```python
from build123d import *

# Parameters (mm, degrees)
F0_W     = 50.4226610065
F0_H     = 49.5728440583
F1_DEPTH = 10
F2_T     = -5
F3_W     = 10.1061211899
F3_H     = 5
F4_DEPTH = 0.5
F7_D     = 1
F7_DEPTH = 2
F7_TIP   = 0.3004303095
F8_R     = 5
F9_R     = 5


# Not quite as in the source:
# - a feature names something its author has since deleted; it is built from what else it names


with BuildPart() as f1:
    # F0 (on Top) → F1 (new body)
    with BuildSketch(Plane.XY):
        Rectangle(F0_W, F0_H)
    extrude(amount=F1_DEPTH)

    # F2
    f2_openings = [f1.faces().sort_by_distance(p)[0] for p in [
        (0, 0, 0),
    ]]
    offset(amount=F2_T, openings=f2_openings)

    # F3 (on face) → F4 (cut)
    with BuildSketch(Plane(origin=(0, 0, 0), x_dir=(1, 0, 0), z_dir=(0, 0, -1))):
        with Locations((-12.4224121682, 22.2864220291)):
            Rectangle(F3_W, F3_H)
    extrude(amount=-F4_DEPTH, mode=Mode.SUBTRACT)

    # F7
    with Locations(Plane(origin=(0, 0, 0.5), x_dir=(1, 0, 0), z_dir=(0, 0, -1))):
        with Locations((-12.5449625775, 22.3620422184)):
            Hole(F7_D / 2, depth=F7_DEPTH)
            with Locations((0, 0, -(F7_DEPTH + F7_TIP / 2))):  # 118° drill point
                Cone(0, F7_D / 2, F7_TIP, mode=Mode.SUBTRACT)

    # F8
    f8_edges = [f1.edges().sort_by_distance(p)[0] for p in [
        (-25.211331, -24.786422, 5),
        (25.211331, -24.786422, 5),
        (25.211331, 24.786422, 5),
        (-25.211331, 24.786422, 5),
    ]]
    fillet(f8_edges, radius=F8_R)

    # F9
    f9_edges = [f1.edges().sort_by_distance(p)[0] for p in [
        (25.211331, 0, 10),
        (23.746864, -23.321956, 10),
        (23.746864, 23.321956, 10),
        (0, -24.786422, 10),
        (0, 24.786422, 10),
        (-23.746864, -23.321956, 10),
        (-23.746864, 23.321956, 10),
        (-25.211331, 0, 10),
    ]]
    fillet(f9_edges, radius=F9_R)


solid = f1.part
```
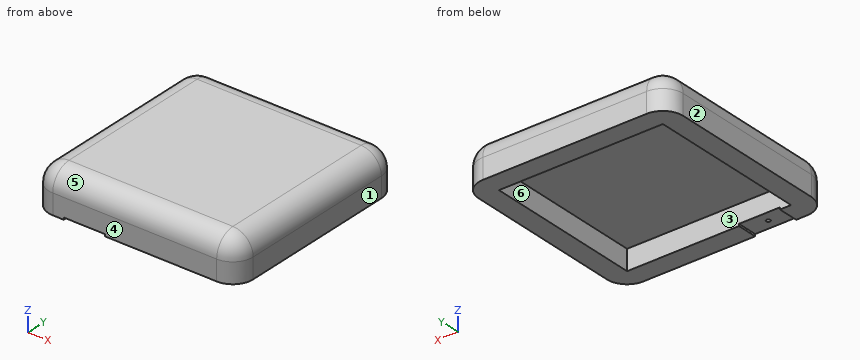
Model file for the job. Use its own axes, mm. Face numbers are marked on the shaded views. A direction names the side the tool comes from. Coordinates: 2 decimals unless noted, no trailing zeros. Order: outer loops, then holes, each group sorted by start corner. A loop starts at its lowest first (then second) coordinate and runs counter-clockwise, first axis right, second up. Notation, with made-up numbers: (75, 35) - (102, 35) arc R22 cw to (102, 43) - close; hole circle Ø9 at (-40, 35.5). An arc over 180 degrees is marked (long way). Return JSON: item names as keys, results as strings. Group by question number.
1) Saw through at D-D, the plane z = 6.25. Write the cut outline in (x, y).
2) Probe line 1 (Y direction, x = -12.5, z = 1); line 2 (X direction, y = 19.5, z = 1.25); line 3 (Y direction, x = 1, z = 2). List the from-to ranges inside material, lowest first. Write a range as from..to.
3) Saw through at C-C, the plane z = 8.75. Write the cut outline in (x, y).
4) Flat gauge pins, fed straight in: P1, Ø2, axis at y = 7.5, z = 8, coming from the +X side; P2, Ø8, axis at x = 1, y = -13, coming from the -Z side; P3, Ø1, axis at x = 19, z = 6.5, coming from the +Y side. Where does each tip first touch, or does it go through?
5) Tool access for the marked faces 5 and 6: list every direction of +Z, -Z, +X, -X, +Y, -Y with a clear straight run to the whole face (end or side of a thin tool).
6) Mould opens along X. For the marked faces 1, 2, 3 and 4 say: released by +X, released by -X, zero draft, split by the parting line, or undercut.
7) Saw through at A-A, the plane y = 5. Write the cut outline in (x, z).
8) Saw through at B-B, the plane x = -15. Write the cut outline in (y, z), plus the area to 3 significant figures.
Values found:
{
 "1": {"outline": "(-25.05, -19.79) arc R4.84 ccw to (-20.21, -24.63) - (20.21, -24.63) arc R4.84 ccw to (25.05, -19.79) - (25.05, 19.79) arc R4.84 ccw to (20.21, 24.63) - (-20.21, 24.63) arc R4.84 ccw to (-25.05, 19.79) - close"},
 "2": {"line 1": "y = -24.79..-22.86, -21.86..-19.79, 19.79..24.79", "line 2": "x = -25.21..-20.21, 20.21..25.21", "line 3": "y = -24.79..-19.79, 19.79..24.79"},
 "3": {"outline": "(-23.52, -19.79) arc R3.31 ccw to (-20.21, -23.09) - (20.21, -23.09) arc R3.31 ccw to (23.52, -19.79) - (23.52, 19.79) arc R3.31 ccw to (20.21, 23.09) - (-20.21, 23.09) arc R3.31 ccw to (-23.52, 19.79) - close"},
 "4": {"P1": "stops at x = 24.79", "P2": "stops at z = 5", "P3": "stops at y = 24.69"},
 "5": {"face 5": "+Z, +X, -X, -Y", "face 6": "-Z"},
 "6": {"face 1": "released by +X", "face 2": "released by -X", "face 3": "undercut", "face 4": "zero draft"},
 "7": {"outline": "(-25.21, 0) - (-20.21, 0) - (-20.21, 5) - (20.21, 5) - (20.21, 0) - (25.21, 0) - (25.21, 5) arc R5 ccw to (20.21, 10) - (-20.21, 10) arc R5 ccw to (-25.21, 5) - close"},
 "8": {"outline": "(-24.79, 0.5) - (-19.79, 0.5) - (-19.79, 5) - (19.79, 5) - (19.79, 0) - (24.79, 0) - (24.79, 5) arc R5 ccw to (19.79, 10) - (-19.79, 10) arc R5 ccw to (-24.79, 5) - close", "area": "285 mm²"}
}
